Autodesk Fusion 360 part; units mm, degrees
sketch "Sketch1" plane through (0, 0, 0) normal (0, 0, 1) x (1, 0, 0)
  circle A0 centre (0, 0) radius 7.5
  line L0 (0, 4) -> (28, 4)
  line L1 (28, 4) -> (28, -4)
  line L2 (28, -4) -> (0, -4)
  line L3 (0, -4) -> (0, 4)
  circle A1 centre (0, 0) radius 1.5
  circle A2 centre (24, 0) radius 1.5
  dimension "d1" = 15
  dimension "d2" = 28
  dimension "d3" = 8
  dimension "d4" = 4
  dimension "d5" = 3
  dimension "d6" = 3
  dimension "d7" = 24
extrude "Extrude1" add sketch "Sketch1" along normal blind 6 contours A0 L0 L2 L3 A1 | A0 L0 L1 L2 | A0 L0 L2 L3 A1
fillet "Fillet1" radius 8 2 edges at (6.3443, -4, 3) (6.3443, 4, 3)
fillet "Fillet2" radius 4 2 edges at (28, 4, 3) (28, -4, 3)
chamfer "Chamfer1" distance 1 angle 45 6 edges at (16.9054, -4, 6) (28, 0, 6) (16.9054, 4, 6) (7.1226, 4.4651, 6) (-7.5, 0, 6) (7.1226, -4.4651, 6)
sketch "Sketch2" plane through (0, 0, 0) normal (0, 0, -1) x (1, 0, 0)
  arc A0 (24, -4) -> (24, 4) centre (24, 0) ccw
  line L0 (24, 4) -> (9.8107, 4)
  arc A1 (4.7471, 5.8065) -> (9.8107, 4) centre (9.8107, 12) ccw
  arc A2 (4.7471, 5.8065) -> (4.7471, -5.8065) centre (0, 0) ccw
  arc A3 (9.8107, -4) -> (4.7471, -5.8065) centre (9.8107, -12) ccw
  line L1 (9.8107, -4) -> (24, -4)
  circle A4 centre (24, 0) radius 1.5
  circle A5 centre (0, 0) radius 1.5
  circle A6 centre (0, 0) radius 3
  dimension "d15" = 6
extrude "Extrude2" cut sketch "Sketch2" against normal blind 4 contours A6
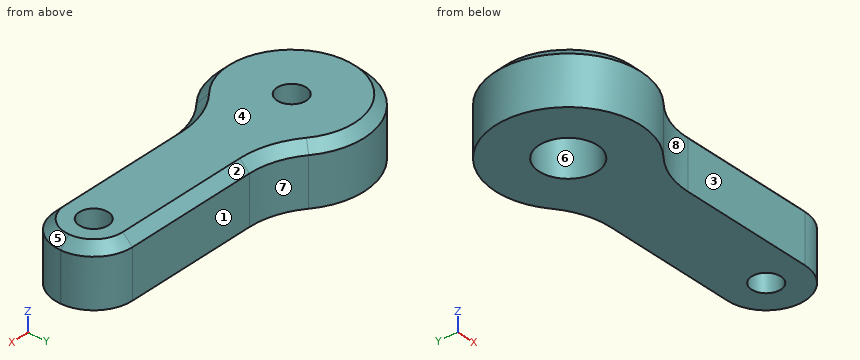
Input: part model. Units: mm. Frame: model coordinates. Face numbers are marked on the shaded views. A direction names the side the tool comes from. Coordinates: 2 decimals unless noted, no trailing zeros. Order: outer loops, then holes, each group sorted by start corner. A loop starts at its lowest first (then second) coordinate and runs counter-clockwise, first axis right, second up. Notation, with made-up numbers: M 58.25,-29.5 L 89.25,-29.5 A18 cw 89.25,0.5 Z; hole C 20.5,67 d8. An arc over 180 degrees is marked long. Answer as CSV lines item,"result".
1. Material intervals for line 1 (Y direction, x = 0, z = 0.85); line 2 (Y direction, x = 24, z = 2.5); line 3 (X direction, y = 1.75, z = 3.75), sorted ascending. Write a range as from..to.
Reported:
line 1,"-7.5..-3, 3..7.5"
line 2,"-4..-1.5, 1.5..4"
line 3,"-7.29..-2.44, 2.44..27.6"
2. Pull-direction query (Y, two-part tool) for the marked faces 6, 7 and 8; classes: released by +Y, released by -Y, zero draft, split by the parting line, or undercut.
Reported:
face 6,"undercut"
face 7,"released by +Y"
face 8,"released by -Y"
3. Section B-B (z = 2.25). State how many separate pieces and enclosed holes the cut face has, then the cut area to 3 significant figures.
Reported:
separate pieces,"1"
enclosed holes,"2"
area,"304 mm2"
4. Section C-C (x = 21.5). Return the cut outline in (y, z), then the cut area to 3 significant figures.
Reported:
outline,"M -4,0 L 4,0 L 4,5 L 3,6 L -3,6 L -4,5 Z"
area,"47.0 mm2"
5. Section A-A (x = 0). Return the cut outline in (y, z).
Reported:
outline,"M -7.5,0 L -3,0 L -3,4 L -1.5,4 L -1.5,6 L -6.5,6 L -7.5,5 Z; M 1.5,4 L 3,4 L 3,0 L 7.5,0 L 7.5,5 L 6.5,6 L 1.5,6 Z"
6. First-contact query: P1, Ø4, axis at x = 16.5, y = 5.5, coming from the +Z side; P2, Ø2.5, axis at x = 17.5, z = 2, coming from the +Y side; P3, Ø5, axis at x = 1.5, y = 0, coming from the -Z side; P4, Ø2.5, axis at x = 14.5, z = 2.5, coming from the -Y side. Flat tips, straight axial feed; report the tip coordinate or a pass-through.
Reported:
P1,"z = 5.5"
P2,"y = 4"
P3,"z = 0"
P4,"y = -4"
7. Access query for the marked faces 1, 2, 3, 4 and 5. Directions: +Z, -Z, +X, -X, +Y, -Y. A direction counts if a zero-diameter tool reaches every point of the face in a straight line with its end or side. Return the directions, or none.
Reported:
face 1,"+Z, -Z, +X, +Y"
face 2,"+Z, +X, +Y"
face 3,"+Z, -Z, +X, -Y"
face 4,"+Z, +X, -X, +Y, -Y"
face 5,"+Z, +X, -Y"
